Source: CAD feature listing. Evaluate the final solid. Frame: model axes, mm. Give positions to 0.01 mm unless a question says otherwise; leave off trailing zeros. Order: outer loops, then holes, each group sorted by start corner. A loop starts at its lowest first (then second) coordinate and runs counter-clockwise, first axis right, second up. Notation, with made-up numbers: (65.5, 76) - (72.5, 76) arc R22 ccw to (72.5, 112) - close; hole circle Ø3 at (65, 9). An arc over 180 degrees is marked (long way). Answer as CSV lines item,"result".
```python
from build123d import *

# Parameters (mm, degrees)
BOSS_EXTRUDE1_DEPTH = 5
SKETCH2_R           = 80
CUT_EXTRUDE5_DEPTH  = 10
SKETCH3_R           = 3
CUT_EXTRUDE6_DEPTH  = 235.360832905


with BuildPart() as part:
    # Lid case → Boss-Extrude1 (new body)
    with BuildSketch(Plane(origin=(0, 0, 0), x_dir=(1, 0, 0), z_dir=(0, 1, 0))):
        with BuildLine():
            Line((-130, 150), (130, 150))
            ThreePointArc((130, 150), (180, 0), (130, -150))
            Line((130, -150), (-130, -150))
            ThreePointArc((-130, -150), (-180, 0), (-130, 150))
        make_face()
    extrude(amount=BOSS_EXTRUDE1_DEPTH)

    # Sketch2 → Cut-Extrude5 (cut)
    with BuildSketch(Plane.XZ):
        with Locations(Location((0, 0, 0), (0, 0, 270))):
            Circle(SKETCH2_R)
    extrude(amount=-CUT_EXTRUDE5_DEPTH, mode=Mode.SUBTRACT)

    # Sketch3 → Cut-Extrude6 (cut, through all)
    with BuildSketch(Plane(origin=(0, 5, 0), x_dir=(1, 0, 0), z_dir=(0, 1, 0))):
        with Locations(Location((-110, 139, 0), (0, 0, 270))):
            Circle(SKETCH3_R)
        with Locations(Location((-82, 139, 0), (0, 0, 270))):
            Circle(SKETCH3_R)
        with Locations(Location((-54, 139, 0), (0, 0, 270))):
            Circle(SKETCH3_R)
        with Locations(Location((54, 139, 0), (0, 0, 270))):
            Circle(SKETCH3_R)
        with Locations(Location((82, 139, 0), (0, 0, 270))):
            Circle(SKETCH3_R)
        with Locations(Location((110, 139, 0), (0, 0, 270))):
            Circle(SKETCH3_R)
    extrude(amount=-CUT_EXTRUDE6_DEPTH, mode=Mode.SUBTRACT)


solid = part.part
```
(1) Ray query, line 1 (X direction, y = 1.7, z = 0); line 2 (X direction, y = 2.4, z = -17); line 3 (Z direction, x = 40.5, y = 2.75). Return the intervals inside material, ascending. Write a range as from..to.
Completed:
line 1,"-180..-80, 80..180"
line 2,"-179.42..-78.17, 78.17..179.42"
line 3,"-150..-68.99, 68.99..150"
(2) Cut plane A-A (x = 0). Return loops of the section in (y, z).
Completed:
outline,"(0, -150) - (5, -150) - (5, -80) - (0, -80) - close; (0, 80) - (5, 80) - (5, 150) - (0, 150) - close"
(3) Cut plane B-B (z = 0). Return loops of the section in (x, y).
Completed:
outline,"(-180, 0) - (-80, 0) - (-80, 5) - (-180, 5) - close; (80, 0) - (180, 0) - (180, 5) - (80, 5) - close"
(4) Contact query for flat-ended pins moving along their axis: pin 1 (5 mm diameter, centred on x = -110, z = -139, fed in from +Y); pin 2 (1 mm diameter, centred on y = 2, z = -20.5, fed in from -X); pin 3 (8 mm diameter, centred on x = 54, z = -139, fed in from -Y); pin 4 (1.5 mm diameter, centred on y = 1, z = -77, fed in from +X). Output: stop coordinate, or through.
Completed:
pin 1,"through"
pin 2,"x = -179.2"
pin 3,"y = 0"
pin 4,"x = 168.09"
(5) Cut plane C-C (y = 2.7). Return loops of the section in (x, z), then the cut area to 3 significant figures.
Completed:
outline,"(-130, -150) - (130, -150) arc R250 ccw to (130, 150) - (-130, 150) arc R250 ccw to start; hole circle Ø6 at (-110, -139); hole circle Ø6 at (-82, -139); hole circle Ø160 at (0, 0); hole circle Ø6 at (-54, -139); hole circle Ø6 at (54, -139); hole circle Ø6 at (82, -139); hole circle Ø6 at (110, -139)"
area,"78,200 mm²"
(6) Mould query, pull axis Z, two halves, no side actions, for faces 1 (the cylindrical face through (-78.1, 2.46, 17.34)), 2 (the flat face through (43, 0, -69)), 3 (the cylindrical face through (179.99, 2.46, -2.25)). Classes: released by +Z, released by -Z, zero draft, split by the parting line, or undercut.
Completed:
face 1,"undercut"
face 2,"zero draft"
face 3,"split by the parting line"
